from build123d import *

# Parameters (mm, degrees)
SKETCH1_R                = 20.55
SKETCH1_R_2              = 1
SKETCH1_W                = 3.1
SKETCH1_H                = 10.1
BASE_FLANGE1_DEPTH       = 2
FILLET1_R                = 10
M4_CLEARANCE_HOLE2_D     = 4.3
M4_CLEARANCE_HOLE2_DEPTH = 136
M4_CLEARANCE_HOLE2_TIP   = 1.291850331


# Sheet-metal steps are written as plain solids
with BuildPart() as part:
    # Sketch1 → Base-Flange1 (new body)
    with BuildSketch(Plane(origin=(0, 0, 0), x_dir=(1, 0, 0), z_dir=(0, 1, 0))):
        with BuildLine():
            Line((-130, -50), (-130, 50))
            Line((-130, 50), (-2.300894967, 59.823008079))
            ThreePointArc((-2.300894967, 59.823008079), (0, 59.911373514), (2.300894967, 59.823008079))
            Line((2.300894967, 59.823008079), (130, 50))
            Line((130, 50), (130, -50))
            Line((130, -50), (7.067672556, -64.582279284))
            ThreePointArc((7.067672556, -64.582279284), (0, -65), (-7.067672556, -64.582279284))
            Line((-7.067672556, -64.582279284), (-130, -50))
        make_face()
        with Locations(Location((0, 0, 0), (0, 0, 270))):
            Circle(SKETCH1_R, mode=Mode.SUBTRACT)
        with Locations(Location((0, 27, 0), (0, 0, 270))):
            Circle(SKETCH1_R_2, mode=Mode.SUBTRACT)
        with Locations(Location((-80.5, 25.5, 0), (0, 0, 270))):
            Circle(SKETCH1_R_2, mode=Mode.SUBTRACT)
        with Locations(Location((-80.5, 4.75, 0), (0, 0, 270))):
            Circle(SKETCH1_R_2, mode=Mode.SUBTRACT)
        with Locations(Location((-80.5, -16, 0), (0, 0, 270))):
            Circle(SKETCH1_R_2, mode=Mode.SUBTRACT)
        with Locations(Location((80.5, -16, 0), (0, 0, 90))):
            Circle(SKETCH1_R_2, mode=Mode.SUBTRACT)
        with Locations(Location((80.5, 4.75, 0), (0, 0, 90))):
            Circle(SKETCH1_R_2, mode=Mode.SUBTRACT)
        with Locations(Location((80.5, 25.5, 0), (0, 0, 90))):
            Circle(SKETCH1_R_2, mode=Mode.SUBTRACT)
        with Locations(Location((27, 0, 0), (0, 0, 270))):
            Circle(SKETCH1_R_2, mode=Mode.SUBTRACT)
        with Locations(Location((0, -27, 0), (0, 0, 270))):
            Circle(SKETCH1_R_2, mode=Mode.SUBTRACT)
        with Locations(Location((-27, 0, 0), (0, 0, 270))):
            Circle(SKETCH1_R_2, mode=Mode.SUBTRACT)
        with Locations(Location((20, -40, 0), (0, 0, 270))):
            Circle(SKETCH1_R_2, mode=Mode.SUBTRACT)
        with Locations(Location((-20, -40, 0), (0, 0, 270))):
            Circle(SKETCH1_R_2, mode=Mode.SUBTRACT)
        with Locations((-61.5, 42)):
            Rectangle(SKETCH1_W, SKETCH1_H, mode=Mode.SUBTRACT)
        with Locations((-61.5, -32.5)):
            Rectangle(SKETCH1_W, SKETCH1_H, mode=Mode.SUBTRACT)
        with Locations((61.5, -32.5)):
            Rectangle(SKETCH1_W, SKETCH1_H, mode=Mode.SUBTRACT)
        with Locations((61.5, 42)):
            Rectangle(SKETCH1_W, SKETCH1_H, mode=Mode.SUBTRACT)
        with BuildLine():
            Line((-120, 39), (-100, 39))
            ThreePointArc((-100, 39), (-96, 35), (-100, 31))
            Line((-100, 31), (-120, 31))
            ThreePointArc((-120, 31), (-124, 35), (-120, 39))
        make_face(mode=Mode.SUBTRACT)
        with BuildLine():
            Line((120, 39), (100, 39))
            ThreePointArc((100, 39), (96, 35), (100, 31))
            Line((100, 31), (120, 31))
            ThreePointArc((120, 31), (124, 35), (120, 39))
        make_face(mode=Mode.SUBTRACT)
        with BuildLine():
            Line((120, -39), (100, -39))
            ThreePointArc((100, -39), (96, -35), (100, -31))
            Line((100, -31), (120, -31))
            ThreePointArc((120, -31), (124, -35), (120, -39))
        make_face(mode=Mode.SUBTRACT)
        with BuildLine():
            Line((-120, -39), (-100, -39))
            ThreePointArc((-100, -39), (-96, -35), (-100, -31))
            Line((-100, -31), (-120, -31))
            ThreePointArc((-120, -31), (-124, -35), (-120, -39))
        make_face(mode=Mode.SUBTRACT)
    extrude(amount=-BASE_FLANGE1_DEPTH)

    # Fillet1
    fillet1_edges = [part.edges().sort_by_distance(p)[0] for p in [
        (130, -1, -50),
        (130, -1, 50),
        (-130, -1, 50),
        (-130, -1, -50),
    ]]
    fillet(fillet1_edges, radius=FILLET1_R)

    # M4 Clearance Hole2
    with Locations(Plane(origin=(0, 0, 0), x_dir=(1, 0, 0), z_dir=(0, 1, 0))):
        with Locations((-27, 0), (0, 27), (27, 0), (0, -27), (20, -40), (-20, -40), (80.5, -16), (80.5, 25.5), (80.5, 4.75), (-80.5, 25.5), (-80.5, 4.75), (-80.5, -16)):
            Hole(M4_CLEARANCE_HOLE2_D / 2, depth=M4_CLEARANCE_HOLE2_DEPTH)
            with Locations((0, 0, -(M4_CLEARANCE_HOLE2_DEPTH + M4_CLEARANCE_HOLE2_TIP / 2))):  # 118° drill point
                Cone(0, M4_CLEARANCE_HOLE2_D / 2, M4_CLEARANCE_HOLE2_TIP, mode=Mode.SUBTRACT)


solid = part.part
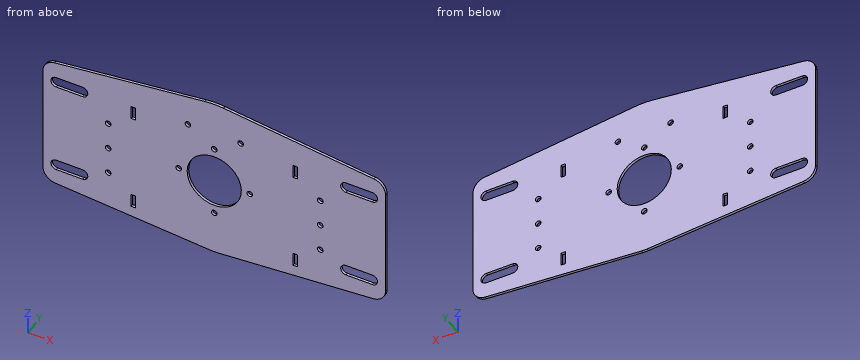
Here's how the part is built. I have some questions about the finished solid (model axes, mm). Coordinates: 2 decimals unless noted, no trailing zeros. Order: outer loops, then holes, each group sorted by start corner. A loop starts at its lowest first (then second) coordinate and runs counter-clockwise, first axis right, second up. Notation, with made-up numbers: (-0.5, 67) - (26.5, 67) arc R37 ccw to (26.5, 105) - close; hole circle Ø3 at (82, -3). An arc over 180 degrees is marked (long way). Use CSV: the item, a comma, the result in double quotes. Start each with the question number.
1. I'm going to push flat-ended pins straight in: pin 1 (1 mm diameter, centred on x = 106.5, y = -1, fed in from -Z); pin 2 (0.6 mm diameter, centred on x = -62, y = -1, fed in from +Z); pin 3 (1 mm diameter, centred on x = -106, y = -1, fed in from -Z); pin 4 (5.5 mm diameter, centred on x = -80.5, z = -4.75, fed in from -Y). Where does each tip first touch, or does it pass through?
2. Suppose I cut it at B-B on x = 13. List the corners of the cut face in (y, z) for me, then the cut area to 3 significant figures.
3. Please list where these lines run through material, in increasing order: line 1 (Z direction, x = -110, y = -1.35); line 2 (X direction, y = -0.35, z = 27); line 3 (X direction, y = -1.5, z = -25.5). Write a range as from..to.
4. Suppose I cut it at A-A on z = 35. List the corners of the cut face in (x, y) for me.
5. Suppose I cut it at C-C on y = -0.9. Give the number of separate pieces and of enclosed holes in the cut face, then the cut area to 3 significant figures.
6. Suppose I cut it at D-D on x = -90. List the corners of the cut face in (y, z) for me, then the cut area to 3 significant figures.
Output:
1,pin 1,"stops at z = -51.85"
1,pin 2,"stops at z = 58.1"
1,pin 3,"stops at z = -51.88"
1,pin 4,"stops at y = -2"
2,outline,"(-2, -59) - (0, -59) - (0, -15.92) - (-2, -15.92) - close; (-2, 15.92) - (0, 15.92) - (0, 63.88) - (-2, 63.88) - close"
2,area,"182 mm2"
3,line 1,"z = -51.54..-39, -31..31, 39..52.37"
3,line 2,"x = -130..-2.15, 2.15..130"
3,line 3,"x = -130..-82.65, -78.35..-1.54, 1.54..78.35, 82.65..130"
4,outline,"(-130, -2) - (-124, -2) - (-124, 0) - (-130, 0) - close; (-96, -2) - (-63.05, -2) - (-63.05, 0) - (-96, 0) - close; (-59.95, -2) - (59.95, -2) - (59.95, 0) - (-59.95, 0) - close; (63.05, -2) - (96, -2) - (96, 0) - (63.05, 0) - close; (124, -2) - (130, -2) - (130, 0) - (124, 0) - close"
5,separate pieces,"1"
5,enclosed holes,"21"
5,area,"26,800 mm2"
6,outline,"(-2, -53.08) - (0, -53.08) - (0, 54.74) - (-2, 54.74) - close"
6,area,"216 mm2"
